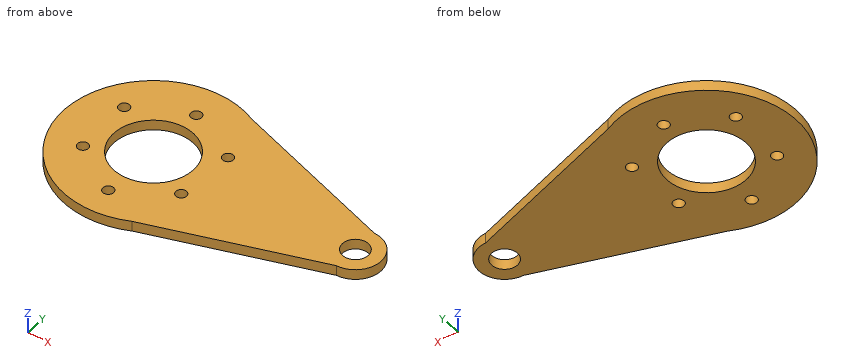
```python
from build123d import *

# Parameters (mm, degrees)
SKETCH_2_R      = 2.1
SKETCH_2_R_2    = 15.5
SKETCH_2_R_3    = 5.03
EXTRUDE_1_DEPTH = 4


with BuildPart() as part:
    # 草图2 → 凸台-拉伸1 (new body)
    with BuildSketch(Plane.XY):
        with BuildLine():
            Line((82.574074367, 4.472412166), (17.886574367, 25.945056537))
            ThreePointArc((17.886574367, 25.945056537), (-32.425925633, -5.527587834), (17.886574367, -37.000232206))
            Line((17.886574367, -37.000232206), (82.574074367, -15.527587834))
            ThreePointArc((82.574074367, -15.527587834), (92.574074367, -5.527587834), (82.574074367, 4.472412166))
        make_face()
        with Locations((2.574074367, -29.277587834)):
            Circle(SKETCH_2_R, mode=Mode.SUBTRACT)
        with Locations((22.059645952, -16.777587834)):
            Circle(SKETCH_2_R, mode=Mode.SUBTRACT)
        with Locations((2.574074367, -5.527587834)):
            Circle(SKETCH_2_R_2, mode=Mode.SUBTRACT)
        with Locations((82.574074367, -5.527587834)):
            Circle(SKETCH_2_R_3, mode=Mode.SUBTRACT)
        with Locations((-17.994028973, 6.347412166)):
            Circle(SKETCH_2_R, mode=Mode.SUBTRACT)
        with Locations((23.142177707, 6.347412166)):
            Circle(SKETCH_2_R, mode=Mode.SUBTRACT)
        with Locations((2.574074367, 16.972412166)):
            Circle(SKETCH_2_R, mode=Mode.SUBTRACT)
        with Locations((-16.911497218, -16.777587834)):
            Circle(SKETCH_2_R, mode=Mode.SUBTRACT)
    extrude(amount=EXTRUDE_1_DEPTH)


solid = part.part
```
Check sheet for the modelled part. Datum: model origin and axes. Units: mm. Coordinates: 2 decimals unless noted, no trailing zeros. Loops run counter-clockwise (first coordinate to the right, second up) from the corner with the lowest first, then second, coordinate; pieces in that order, holes last. Notation, with made-up numbers: M -31.5,57.5 L 8.5,57.5 A15 ccw 8.5,80.5 Z; hole C 68,65 d2. An arc over 180 degrees is marked long. Answer as a JSON object with one key per item and string values.
1. Sectioned sample at D-D on x = 63.5. Record the cut outline in (y, z), and give its area (3 significant figures).
Outcome:
{"outline": "M -21.86,0 L 10.8,0 L 10.8,4 L -21.86,4 Z", "area": "131 mm²"}
2. Depth check by flat-ended pin: P1, Ø2.5, axis at x = 2.57, y = 16.97, coming from the -Z side. Enter the tip coordinate at first touch or a pass-through.
Outcome:
{"P1": "through"}
3. Sectioned sample at C-C on z = 1.7. Count the separate pieces of the cut face and the enclosed holes in it, and give its area (3 significant figures).
Outcome:
{"separate pieces": "1", "enclosed holes": "8", "area": "4,880 mm²"}
4. Scan lines: L1, parallel to X at y = -4, z = 0.7; L2, parallel to Y at x = -16.5, z = 2.9; L3, parallel to X at y = -6.5, z = 0.9. Record each from-to range of solid material in increasing order. Write a range as from..to.
Outcome:
{"L1": "-32.39..-12.85, 18..77.78, 87.37..92.46", "L2": "-34.87..-18.84, -14.72..4.87, 7.82..23.82", "L3": "-32.41..-12.9, 18.04..77.64, 87.51..92.53"}
5. Sectioned sample at A-A on x = -11. Record the cut outline in (y, z).
Outcome:
{"outline": "M -37.79,0 L -13.01,0 L -13.01,4 L -37.79,4 Z; M 1.96,0 L 26.73,0 L 26.73,4 L 1.96,4 Z"}
6. Sectioned sample at B-B on y = 1.5. Record the cut outline in (x, z).
Outcome:
{"outline": "M -31.71,0 L -11.24,0 L -11.24,4 L -31.71,4 Z; M 16.39,0 L 89.69,0 L 89.69,4 L 16.39,4 Z"}
